from build123d import *

# Parameters (mm, degrees)
SKETCH_1_R          = 2.1
EXTRUDE_1_DEPTH     = 2
SKETCH_3_R          = 2.1
CUT_EXTRUDE_2_DEPTH = 10


with BuildPart() as part:
    # Эскиз1 → Бобышка-Вытянуть1 (new body)
    with BuildSketch(Plane.XY):
        with BuildLine():
            Line((-7.5, 173), (-7.5, -3))
            ThreePointArc((-7.5, -3), (-6.914213562, -4.414213562), (-5.5, -5))
            Line((-5.5, -5), (5.5, -5))
            ThreePointArc((5.5, -5), (6.914213562, -4.414213562), (7.5, -3))
            Line((7.5, -3), (7.5, 173))
            ThreePointArc((7.5, 173), (6.914213562, 174.414213562), (5.5, 175))
            Line((5.5, 175), (-5.5, 175))
            ThreePointArc((-5.5, 175), (-6.914213562, 174.414213562), (-7.5, 173))
        make_face()
        with Locations((0, 170)):
            Circle(SKETCH_1_R, mode=Mode.SUBTRACT)
        with Locations((0, 150)):
            Circle(SKETCH_1_R, mode=Mode.SUBTRACT)
        with Locations((0, 20)):
            Circle(SKETCH_1_R, mode=Mode.SUBTRACT)
        Circle(SKETCH_1_R, mode=Mode.SUBTRACT)
    extrude(amount=EXTRUDE_1_DEPTH)

    # Эскиз3 → Вырез-Вытянуть2 (cut)
    with BuildSketch(Plane.XY.offset(2)):
        with Locations((0, 45)):
            Circle(SKETCH_3_R)
    extrude(amount=-CUT_EXTRUDE_2_DEPTH, mode=Mode.SUBTRACT)


solid = part.part
Source: CAD feature listing. Evaluate the final solid. Frame: model axes, mm. Give positions to 0.01 mm unless a question says otherwise; leave off trailing zeros. Order: outer loops, then holes, each group sorted by start corner. A loop starts at its lowest first (then second) coordinate and runs counter-clockwise, first axis right, second up. Notation, with made-up numbers: (-11, -19.5) -> (25, -19.5) arc R13 ccw to (25, -7.5) -> close; hole circle Ø6 at (33, -3.5). An arc over 180 degrees is marked (long way). Use a Markdown table: item, result.
1) Ray query, line 1 along Y through (x, z) = (0.5, 0.7); line 2 along Y through (x, z) = (-1.75, 1.7); line 3 along X through (y, z) = (149, 1.35). Return the intervals inside material, ascending. Write a range as [from, to].
Answer list:
| item | result |
|---|---|
| line 1 | [-5, -2.04], [2.04, 17.96], [22.04, 42.96], [47.04, 147.96], [152.04, 167.96], [172.04, 175] |
| line 2 | [-5, -1.16], [1.16, 18.84], [21.16, 43.84], [46.16, 148.84], [151.16, 168.84], [171.16, 175] |
| line 3 | [-7.5, -1.85], [1.85, 7.5] |
2) Section query B-B, the plane z = 1.2. Return the cut outline in (x, y).
Answer list:
| item | result |
|---|---|
| outline | (-7.5, -3) arc R2 ccw to (-5.5, -5) -> (5.5, -5) arc R2 ccw to (7.5, -3) -> (7.5, 173) arc R2 ccw to (5.5, 175) -> (-5.5, 175) arc R2 ccw to (-7.5, 173) -> close; hole circle Ø4.2 at (0, 0); hole circle Ø4.2 at (0, 20); hole circle Ø4.2 at (0, 45); hole circle Ø4.2 at (0, 150); hole circle Ø4.2 at (0, 170) |
3) Mould query, pull axis Y, two halves, no side actions, for faces 1 (the flat face through (0, 86, 2)), 2 (the cylindrical face through (-0.46, 42.95, 1.01)). Classes: +Y half, -Y half, draft (parallel to the pull), parting line (faces both ways), or undercut.
Answer list:
| item | result |
|---|---|
| face 1 | draft |
| face 2 | undercut |
4) Contact query for a flat-ended pin moving along its axis: P1, Ø3.5, axis at x = 0, y = 170, coming from the +Z side. Output: stop coordinate, or through.
Answer list:
| item | result |
|---|---|
| P1 | through |
5) Section query C-C, the plane x = 0.5. Return the cut outline in (y, z).
Answer list:
| item | result |
|---|---|
| outline | (-5, 0) -> (-2.04, 0) -> (-2.04, 2) -> (-5, 2) -> close; (2.04, 0) -> (17.96, 0) -> (17.96, 2) -> (2.04, 2) -> close; (22.04, 0) -> (42.96, 0) -> (42.96, 2) -> (22.04, 2) -> close; (47.04, 0) -> (147.96, 0) -> (147.96, 2) -> (47.04, 2) -> close; (152.04, 0) -> (167.96, 0) -> (167.96, 2) -> (152.04, 2) -> close; (172.04, 0) -> (175, 0) -> (175, 2) -> (172.04, 2) -> close |
6) Section query A-A, the plane y = 0. Return the cut outline in (x, z).
Answer list:
| item | result |
|---|---|
| outline | (-7.5, 0) -> (-2.1, 0) -> (-2.1, 2) -> (-7.5, 2) -> close; (2.1, 0) -> (7.5, 0) -> (7.5, 2) -> (2.1, 2) -> close |
